Read the model definition and answer for the solid it produces. Units are mm, in the model's axes. A direction names the side the tool comes from. Coordinates: 2 decimals unless noted, no trailing zeros. Loops run counter-clockwise (first coordinate to the right, second up) from the corner with the lowest first, then second, coordinate; pieces in that order, holes last.
from build123d import *

# Parameters (mm, degrees)
PAD005_DEPTH    = 3
SKETCH009_W     = 3.3
SKETCH009_H     = 3.3
POCKET003_DEPTH = 3.001
CHAMFER001_SIZE = 0.25
CHAMFER004_SIZE = 0.25
CHAMFER007_SIZE = 0.25


with BuildPart() as part:
    # Sketch008 → Pad005 (new body)
    with BuildSketch(Plane.XY):
        with BuildLine():
            Line((-36.502214, 3.5), (36.502214, 3.5))
            ThreePointArc((38.502214, 1.5), (37.916428, 2.914214), (36.502214, 3.5))
            Line((38.502214, 1.5), (38.502214, -1.5))
            ThreePointArc((36.502214, -3.5), (37.916428, -2.914214), (38.502214, -1.5))
            Line((36.502214, -3.5), (-36.502214, -3.5))
            ThreePointArc((-38.502214, -1.5), (-37.916428, -2.914214), (-36.502214, -3.5))
            Line((-38.502214, -1.5), (-38.502214, 1.5))
            ThreePointArc((-36.502214, 3.5), (-37.916428, 2.914214), (-38.502214, 1.5))
        make_face()
    extrude(amount=PAD005_DEPTH)

    # Sketch009 → Pocket003 (cut, through all)
    with BuildSketch(Plane.XY.offset(3)):
        with Locations((-6, 0)):
            Rectangle(SKETCH009_W, SKETCH009_H)
        with Locations((10.7, 0)):
            Rectangle(SKETCH009_W, SKETCH009_H)
    extrude(amount=-POCKET003_DEPTH, mode=Mode.SUBTRACT)

    # Chamfer001
    chamfer001_edges = [part.edges().sort_by_distance(p)[0] for p in [
        (0, -3.5, 3),
        (0, 3.5, 3),
    ]]
    chamfer(chamfer001_edges, length=CHAMFER001_SIZE)

    # Chamfer004
    chamfer004_edges = [part.edges().sort_by_distance(p)[0] for p in [
        (-7.65, 0, 0),
        (-6, 1.65, 0),
        (-4.35, 0, 0),
        (-6, -1.65, 0),
        (9.05, 0, 0),
        (10.7, -1.65, 0),
        (12.35, 0, 0),
        (10.7, 1.65, 0),
    ]]
    chamfer(chamfer004_edges, length=CHAMFER004_SIZE)

    # Chamfer007
    chamfer007_edges = [part.edges().sort_by_distance(p)[0] for p in [
        (9.05, 0, 3),
        (10.7, 1.65, 3),
        (12.35, 0, 3),
        (10.7, -1.65, 3),
        (-4.35, 0, 3),
        (-6, -1.65, 3),
        (-7.65, 0, 3),
        (-6, 1.65, 3),
    ]]
    chamfer(chamfer007_edges, length=CHAMFER007_SIZE)


solid = part.part
Q1. Determine the mould class of faces 1 (the face through (-37.93, -2.9, 1.36)), 2 (the face through (12.35, 0, 2)), 3 (the face through (-7.65, 0, 2)), 4 (the face through (1, -3.5, 1)) for opening direction X: +X half, -X half, draft (parallel to the pull), parting line (faces both ways), or undercut.
Findings below:
face 1: -X half
face 2: undercut
face 3: undercut
face 4: draft
Q2. A cutting plane is placed at B-B (x = -7). Give the vertices of the cut face in (y, z), then the cut area to 3 significant figures.
Findings below:
outline: (-3.5, 0) - (-1.9, 0) - (-1.65, 0.25) - (-1.65, 2.75) - (-1.9, 3) - (-3.25, 3) - (-3.5, 2.75) - close; (1.65, 0.25) - (1.9, 0) - (3.5, 0) - (3.5, 2.75) - (3.25, 3) - (1.9, 3) - (1.65, 2.75) - close
area: 10.9 mm2
Q3. Straight lines are drawn through the part: probe 1 along X at (y, z) = (-1.5, 2.5); probe 2 along X at (y, z) = (1, 2.8); probe 3 along Y at (x, z) = (10.5, 2.85). For each, find the intervals that lie inside material, in ascending order.
Findings below:
probe 1: x = -38.5 to -7.65, -4.35 to 9.05, 12.35 to 38.5
probe 2: x = -38.45 to -7.7, -4.3 to 9, 12.4 to 38.45
probe 3: y = -3.4 to -1.75, 1.75 to 3.4
Q4. A cutting plane is placed at A-A (y = 0.5). Give the vertices of the cut face in (x, z).
Findings below:
outline: (-38.5, 0) - (-7.9, 0) - (-7.65, 0.25) - (-7.65, 2.75) - (-7.9, 3) - (-38.25, 3) - (-38.5, 2.75) - close; (-4.35, 0.25) - (-4.1, 0) - (8.8, 0) - (9.05, 0.25) - (9.05, 2.75) - (8.8, 3) - (-4.1, 3) - (-4.35, 2.75) - close; (12.35, 0.25) - (12.6, 0) - (38.5, 0) - (38.5, 2.75) - (38.25, 3) - (12.6, 3) - (12.35, 2.75) - close
Q5. A cutting plane is placed at C-C (z = 1.65). Give the vertices of the cut face in (x, y), then the cut area to 3 significant figures.
Findings below:
outline: (-38.5, -1.5) arc R2 ccw to (-36.5, -3.5) - (36.5, -3.5) arc R2 ccw to (38.5, -1.5) - (38.5, 1.5) arc R2 ccw to (36.5, 3.5) - (-36.5, 3.5) arc R2 ccw to (-38.5, 1.5) - close; hole (-7.65, -1.65) - (-4.35, -1.65) - (-4.35, 1.65) - (-7.65, 1.65) - close; hole (9.05, -1.65) - (12.35, -1.65) - (12.35, 1.65) - (9.05, 1.65) - close
area: 514 mm2
Q6. Which of the six approach directions +Z, -Z, +X, -X, +Y, -Y give full straight-line access (tool end or side, diameter ignored) to faces 5 (the face through (-6, 1.65, 2)), 6 (the face through (-37.844, 2.812, 2.873))?
Findings below:
face 5: +Z, -Z
face 6: +Z, -X, +Y
